Job drawing, mm, ordinate dimensions from the low corner. One solid piece. A direction names the side the tool comes from. Round coordinates to 2 decimals unless told otherwise and drop trailing zeros. Loops run counter-clockwise (first coordinate to the right, second up) from the corner with the lowest first, then second, coordinate; pieces in that order, holes last. Notation, with made-up numbers: (-37, 45.5) - (-7, 45.5) arc R24 cw to (-7, 82.5) - close; hole circle Ø2 at (64.25, 12.25). An arc over 180 degrees is marked (long way). Answer as CSV lines item,"result". Start each with the question number.
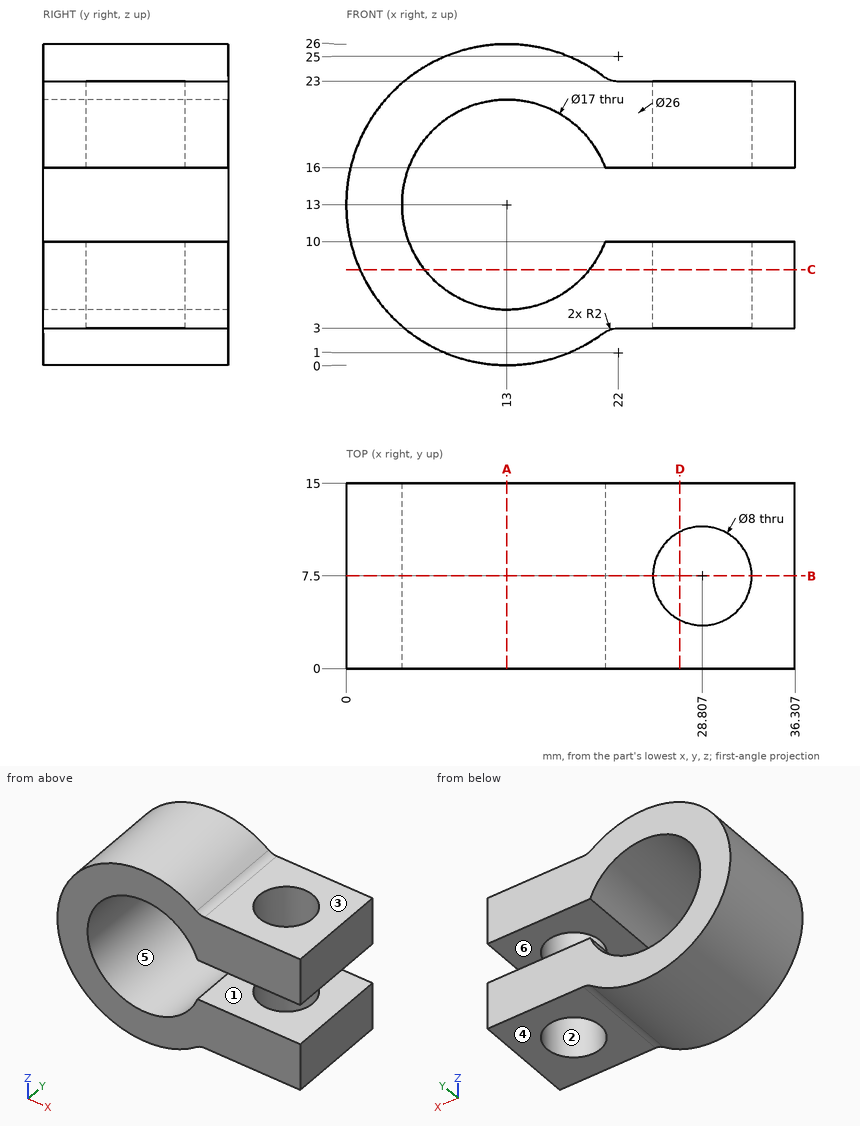
Q1. Band-saw the part on B-B, the plane y = 7.5. List the corners of the cut face in (x, z).
Q2. Band-saw the part on C-C, the plane z = 7.75. List the corners of the cut face in (x, y) (1 decimal), then the cut area to 3 significant figures.
Q3. Band-saw the part on D-D, the plane x = 27. List the corners of the cut face in (y, z).
Q4. Two-plate mould, pull along Z, no slides. Class the marked faces 1, 2 and 3: released by +Z, released by -Z, zero draft, split by the parting line, or undercut.
Q5. Wall check: probe 1 along Z at (x, y) = (30, 11.5); probe 2 along X at (y, z) = (8.5, 18.25) (1 decimal); probe 3 along Z at (x, y) = (13, 5.5). Give the ranges that are in metal, low to high. Write a range as [from, to].
Q6. Tool access for the marked faces 4, 5 and 6: list every direction of +Z, -Z, +X, -X, +Y, -Y with a clear straight run to the whole face (end or side of a thin tool).
Q7. Band-saw the part on A-A, the plane x = 13. List the corners of the cut face in (y, z).
Q8. Pin check, flat tips, straight feed: pin 1 Ø7 at (x, y) = (27, 7) entering from -Z; pin 2 Ø8 at (y, z) = (11.5, 7.5) entering from -X; pin 3 Ø6 at (x, y) = (17, 10) entering from -Z. Stop position of each tip, or through.
Reported:
1,outline,"(20.8, 2.6) arc R2 cw to (22, 3) - (24.81, 3) - (24.81, 10) - (20.95, 10) arc R8.5 cw (long way) to (20.95, 16) - (24.81, 16) - (24.81, 23) - (22, 23) arc R2 cw to (20.8, 23.4) arc R13 ccw (long way) to start; (32.81, 3) - (36.31, 3) - (36.31, 10) - (32.81, 10) - close; (32.81, 16) - (36.31, 16) - (36.31, 23) - (32.81, 23) - close"
2,outline,"(1.1, 0) - (6.3, 0) - (6.3, 15) - (1.1, 15) - close; (19.7, 0) - (36.3, 0) - (36.3, 15) - (19.7, 15) - close; hole circle Ø8 at (28.8, 7.5)"
2,area,"277 mm2"
3,outline,"(0, 3) - (3.93, 3) - (3.93, 10) - (0, 10) - close; (0, 16) - (3.93, 16) - (3.93, 23) - (0, 23) - close; (11.07, 3) - (15, 3) - (15, 10) - (11.07, 10) - close; (11.07, 16) - (15, 16) - (15, 23) - (11.07, 23) - close"
4,face 1,"undercut"
4,face 2,"zero draft"
4,face 3,"released by +Z"
5,probe 1,"z = [3, 10], [16, 23]"
5,probe 2,"x = [1.1, 6.3], [19.7, 24.9], [32.7, 36.3]"
5,probe 3,"z = [0, 4.5], [21.5, 26]"
6,face 4,"-Z, +X, +Y, -Y"
6,face 5,"+Y, -Y"
6,face 6,"+X, +Y, -Y"
7,outline,"(0, 0) - (15, 0) - (15, 4.5) - (0, 4.5) - close; (0, 21.5) - (15, 21.5) - (15, 26) - (0, 26) - close"
8,pin 1,"stops at z = 3"
8,pin 2,"stops at x = 0.09"
8,pin 3,"stops at z = 0.04"
